Geometry check sheet. Reference: the model listing, model coordinates, mm. Face numbers are marked on the shaded views. A direction names the side the tool comes from. Coordinates: 2 decimals unless noted, no trailing zeros. Write each loop counter-clockwise with the first axis right and the second up, starting at its lowest first coordinate (ties: lowest second). Pieces come first, ordered by that corner, then holes.
from build123d import *
from build123d.topology import SkipClean

# Parameters (mm, degrees)
BOSS_EXTRUDE1_DEPTH = 11.1125
SKETCH3_R           = 17.6
BOSS_EXTRUDE2_DEPTH = 12.7
SKETCH3_5_R         = 11.25
CUT_EXTRUDE2_DEPTH  = 7.5
SKETCH3_6_R         = 9
CUT_EXTRUDE3_DEPTH  = 12.7
BOSS_EXTRUDE3_START = -31.9278
BOSS_EXTRUDE3_DEPTH = 4.953
FILLET1_R           = 1.016
SKETCH5_R           = 1.905
CUT_EXTRUDE4_DEPTH  = 96.510603758
FILLET3_R           = 1.016
CUT_EXTRUDE5_START  = -3.175
CUT_EXTRUDE5_DEPTH  = 3.175
SKETCH9_W           = 10.961249955
SKETCH9_H           = 7.9375
CUT_EXTRUDE6_DEPTH  = 3.175
CUT_EXTRUDE9_DEPTH  = 2.54
SKETCH13_R          = 12.7
SKETCH13_R_2        = 9
BOSS_EXTRUDE6_DEPTH = 3.175
CHAMFER2_SIZE       = 3.175
SKETCH15_R          = 2.54
CUT_EXTRUDE10_DEPTH = 91.477679673


with BuildPart() as part:
    # Sketch2 → Boss-Extrude1 (new, symmetric)
    with BuildSketch(Plane(origin=(0, 0, 0), x_dir=(1, 0, 0), z_dir=(0, 1, 0))):
        Polygon((0, 0), (-57.15, 0), (-84.090768363, -26.940768363), (-76.008537854, -35.022998872), (-53.685538982, -12.7), (0, -12.7), align=None)
        Polygon((57.15, 0), (0, 0), (0, -12.7), (53.685538982, -12.7), (76.008537854, -35.022998872), (84.090768363, -26.940768363), align=None)
    extrude(amount=BOSS_EXTRUDE1_DEPTH, both=True)

    # Sketch3 → Boss-Extrude2 (add)
    with BuildSketch(Plane(origin=(0, 0, 0), x_dir=(-1, 0, 0), z_dir=(0, 0, -1))):
        Circle(SKETCH3_R)
    extrude(amount=-BOSS_EXTRUDE2_DEPTH)

    # Sketch3<5> → Cut-Extrude2 (cut)
    with BuildSketch(Plane(origin=(0, 0, 0), x_dir=(-1, 0, 0), z_dir=(0, 0, -1))):
        Circle(SKETCH3_5_R)
    extrude(amount=-CUT_EXTRUDE2_DEPTH, mode=Mode.SUBTRACT)

    # Sketch3<6> → Cut-Extrude3 (cut)
    with BuildSketch(Plane(origin=(0, 0, 0), x_dir=(-1, 0, 0), z_dir=(0, 0, -1))):
        Circle(SKETCH3_6_R)
    extrude(amount=-CUT_EXTRUDE3_DEPTH, mode=Mode.SUBTRACT)

    # Sketch4 → Boss-Extrude3 (add)
    with BuildSketch(Plane(origin=(55.515768363, 0, 55.515768363), x_dir=(0.707106781186549, 0, -0.707106781186546), z_dir=(0.707106781186546, 0, 0.707106781186549)).offset(BOSS_EXTRUDE3_START)):
        Polygon((27.481152545, -12.6125), (40.411152545, -12.6125), (40.411152545, -11.1125), (28.981152545, -11.1125), (28.981152545, 11.1125), (40.411152545, 11.1125), (40.411152545, 12.6125), (27.481152545, 12.6125), align=None)
    boss_extrude3 = extrude(amount=BOSS_EXTRUDE3_DEPTH)

    # Fillet1
    fillet1_edges = [part.edges().sort_by_distance(p)[0] for p in [
        (66.471505854, -11.1125, 25.485966872),
        (66.471505854, 11.1125, 25.485966872),
    ]]
    fillet(fillet1_edges, radius=FILLET1_R)

    # Sketch5 → Cut-Extrude4 (cut, through all)
    with BuildSketch(Plane(origin=(0, 11.1125, 0), x_dir=(1, 0, 0), z_dir=(0, 1, 0))):
        with BuildLine():
            ThreePointArc((73.278539993, -23.851560258), (73.278539993, -26.545637094), (75.97261683, -26.545637094))
            Line((75.97261683, -26.545637094), (73.278539993, -23.851560258))
        make_face()
        with BuildLine():
            Line((73.278539993, -23.851560258), (75.97261683, -26.545637094))
            ThreePointArc((75.97261683, -26.545637094), (76.385568921, -25.927610614), (76.530578412, -25.198598676))
            ThreePointArc((76.530578412, -25.198598676), (75.35459035, -23.438608166), (73.278539993, -23.851560258))
        make_face()
        with Locations(Location((65.645322291, -16.218342555, 0), (0, 0, 270))):
            Circle(SKETCH5_R)
    cut_extrude4 = extrude(amount=-CUT_EXTRUDE4_DEPTH, mode=Mode.SUBTRACT)

    # Mirror2: Boss-Extrude3, Cut-Extrude4 across plane
    add(boss_extrude3.mirror(Plane(origin=(0, 0, 0), x_dir=(0, 0, 1), z_dir=(1, 0, 0))))
    add(cut_extrude4.mirror(Plane(origin=(0, 0, 0), x_dir=(0, 0, 1), z_dir=(1, 0, 0))), mode=Mode.SUBTRACT)

    # Fillet3
    fillet3_edges = [part.edges().sort_by_distance(p)[0] for p in [
        (-66.471505854, -11.1125, 25.485966872),
        (-66.471505854, 11.1125, 25.485966872),
    ]]
    fillet(fillet3_edges, radius=FILLET3_R)

    # Sketch6 → Cut-Extrude5 (cut)
    with BuildSketch(Plane.XY.offset(12.7).offset(CUT_EXTRUDE5_START)):
        with BuildLine():
            Line((-53.17880895, 11.1125), (-53.17880895, 3.175))
            Line((-53.17880895, 3.175), (-17.311249955, 3.175))
            ThreePointArc((-17.311249955, 3.175), (-15.980371829, 7.374802791), (-13.648162651, 11.1125))
            Line((-13.648162651, 11.1125), (-53.17880895, 11.1125))
        make_face()
        with BuildLine():
            Line((-17.311249955, -3.175), (-53.17880895, -3.175))
            Line((-53.17880895, -3.175), (-53.17880895, -11.1125))
            Line((-53.17880895, -11.1125), (-13.648162651, -11.1125))
            ThreePointArc((-13.648162651, -11.1125), (-15.980371829, -7.374802791), (-17.311249955, -3.175))
        make_face()
        with BuildLine():
            Line((53.17880895, 11.1125), (13.648162651, 11.1125))
            ThreePointArc((13.648162651, 11.1125), (15.980371829, 7.374802791), (17.311249955, 3.175))
            Line((17.311249955, 3.175), (53.17880895, 3.175))
            Line((53.17880895, 3.175), (53.17880895, 11.1125))
        make_face()
        with BuildLine():
            ThreePointArc((17.311249955, -3.175), (15.980371829, -7.374802791), (13.648162651, -11.1125))
            Line((13.648162651, -11.1125), (53.17880895, -11.1125))
            Line((53.17880895, -11.1125), (53.17880895, -3.175))
            Line((53.17880895, -3.175), (17.311249955, -3.175))
        make_face()
    extrude(amount=CUT_EXTRUDE5_DEPTH, mode=Mode.SUBTRACT)

    # Sketch9 → Cut-Extrude6 (cut)
    with SkipClean():  # the faces are left unmerged after this step: merging them gives an invalid solid
        with BuildSketch(Plane(origin=(0, 0, 0), x_dir=(-1, 0, 0), z_dir=(0, 0, -1))):
            with Locations((62.630624978, -7.14375)):
                Rectangle(SKETCH9_W, SKETCH9_H)
            with BuildLine():
                ThreePointArc((17.311249955, -3.175), (15.980371829, -7.374802791), (13.648162651, -11.1125))
                Line((13.648162651, -11.1125), (57.15, -11.1125))
                Line((57.15, -11.1125), (57.15, -3.175))
                Line((57.15, -3.175), (17.311249955, -3.175))
            make_face()
            with BuildLine():
                Line((57.15, 11.1125), (13.648162651, 11.1125))
                ThreePointArc((13.648162651, 11.1125), (15.980371829, 7.374802791), (17.311249955, 3.175))
                Line((17.311249955, 3.175), (57.15, 3.175))
                Line((57.15, 3.175), (57.15, 11.1125))
            make_face()
            with Locations((62.630624978, 7.14375)):
                Rectangle(SKETCH9_W, SKETCH9_H)
            with BuildLine():
                ThreePointArc((-13.648162651, -11.1125), (-15.980371829, -7.374802791), (-17.311249955, -3.175))
                Line((-17.311249955, -3.175), (-57.15, -3.175))
                Line((-57.15, -3.175), (-57.15, -11.1125))
                Line((-57.15, -11.1125), (-13.648162651, -11.1125))
            make_face()
            with Locations((-62.630624978, -7.14375)):
                Rectangle(SKETCH9_W, SKETCH9_H)
            with BuildLine():
                Line((-57.15, 3.175), (-17.311249955, 3.175))
                ThreePointArc((-17.311249955, 3.175), (-15.980371829, 7.374802791), (-13.648162651, 11.1125))
                Line((-13.648162651, 11.1125), (-57.15, 11.1125))
                Line((-57.15, 11.1125), (-57.15, 3.175))
            make_face()
            with Locations((-62.630624978, 7.14375)):
                Rectangle(SKETCH9_W, SKETCH9_H)
        extrude(amount=-CUT_EXTRUDE6_DEPTH, mode=Mode.SUBTRACT)

    # Sketch12 → Cut-Extrude9 (cut)
    with SkipClean():  # the faces are left unmerged after this step: merging them gives an invalid solid
        with BuildSketch(Plane(origin=(55.515768363, 0, 55.515768363), x_dir=(0.7071067811865486, 0, -0.7071067811865465), z_dir=(0.7071067811865465, 0, 0.7071067811865486))):
            with BuildLine():
                Line((28.981152545, 10.0965), (28.981152545, -10.0965))
                ThreePointArc((28.981152545, -10.0965), (29.278732055, -10.81492049), (29.997152545, -11.1125))
                Line((29.997152545, -11.1125), (40.411152545, -11.1125))
                Line((40.411152545, -11.1125), (40.411152545, 11.1125))
                Line((40.411152545, 11.1125), (29.997152545, 11.1125))
                ThreePointArc((29.997152545, 11.1125), (29.278732055, 10.81492049), (28.981152545, 10.0965))
            make_face()
        cut_extrude9 = extrude(amount=-CUT_EXTRUDE9_DEPTH, mode=Mode.SUBTRACT)

    # Mirror3: Cut-Extrude9 across plane
    with SkipClean():  # the faces are left unmerged after this step: merging them gives an invalid solid
        add(cut_extrude9.mirror(Plane(origin=(0, 0, 0), x_dir=(0, 0, 1), z_dir=(1, 0, 0))), mode=Mode.SUBTRACT)

    # Sketch13 → Boss-Extrude6 (add)
    with SkipClean():  # the faces are left unmerged after this step: merging them gives an invalid solid
        with BuildSketch(Plane.XY.offset(12.7)):
            Circle(SKETCH13_R)
            with Locations(Location((0, 0, 0), (0, 0, 180))):
                Circle(SKETCH13_R_2, mode=Mode.SUBTRACT)
        extrude(amount=BOSS_EXTRUDE6_DEPTH)

    # Chamfer2
    chamfer2_edges = [part.edges().sort_by_distance(p)[0] for p in [
        (53.17880895, 7.14375, 9.525),
        (53.17880895, -7.14375, 9.525),
        (-53.17880895, 7.14375, 9.525),
        (-53.17880895, -7.14375, 9.525),
    ]]
    chamfer(chamfer2_edges, length=CHAMFER2_SIZE - 0.0001)  # a hair under: the kernel refuses the full size

    # Sketch15 → Cut-Extrude10 (cut, through all)
    with BuildSketch(Plane(origin=(0, 0, 0), x_dir=(-1, 0, 0), z_dir=(0, 0, -1))):
        with Locations((21.59, 0)):
            Circle(SKETCH15_R)
        with Locations(Location((-21.59, 0, 0), (0, 0, 180))):
            Circle(SKETCH15_R)
    extrude(amount=-CUT_EXTRUDE10_DEPTH, mode=Mode.SUBTRACT)


solid = part.part
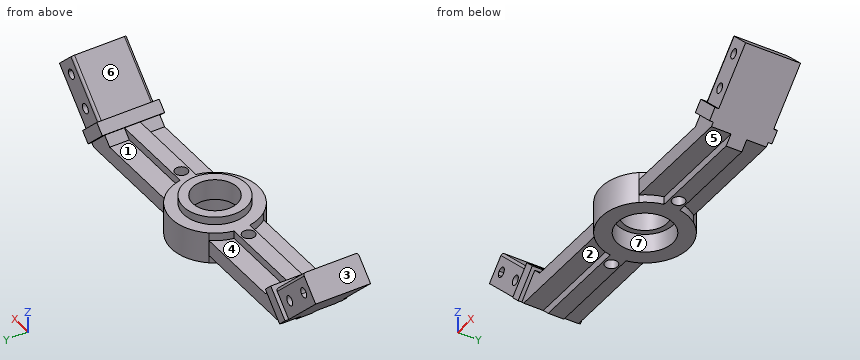
1. Sectioned sample at A-A, the plane x = 21.59. Record the boundary of the cut face in (y, z) (1 decimal), and give its area (3 significant figures).
Computed values:
outline: (-11.1, 3.2) - (-3.2, 3.2) - (-3.2, 0) - (-2.5, 0) - (-2.5, 12.7) - (-3.2, 12.7) - (-3.2, 9.5) - (-11.1, 9.5) - close; (2.5, 0) - (3.2, 0) - (3.2, 3.2) - (11.1, 3.2) - (11.1, 9.5) - (3.2, 9.5) - (3.2, 12.7) - (2.5, 12.7) - close
area: 117 mm2
2. Sectioned sample at D-D, the plane x = 0. Record the boundary of the cut face in (y, z) (3 decimals).
Computed values:
outline: (-17.6, 0) - (-11.25, 0) - (-11.25, 7.5) - (-9, 7.5) - (-9, 15.875) - (-12.7, 15.875) - (-12.7, 12.7) - (-17.6, 12.7) - close; (9, 7.5) - (11.25, 7.5) - (11.25, 0) - (17.6, 0) - (17.6, 12.7) - (12.7, 12.7) - (12.7, 15.875) - (9, 15.875) - close
3. Access from +Z, -Z, +X, -X, +Y, -Y to the whole of each face (thin tool, end or side, straight path). Record for the marked faces 4, 5, 6 and 7.
Computed values:
face 4: +Z, +Y
face 5: -Z, +X, -Y
face 6: +Z, +Y, -Y
face 7: -Z
4. Gauge pin test, flat ends, axial feed: pin 1 Ø8 at (y, z) = (-6.5, 25) entering from +X; pin 2 Ø1.5 at (y, z) = (13, 12.5) entering from +X; pin 3 Ø5 at (x, z) = (38, 10) entering from -Y. Record the tip position at first contact, or that the pin passes through.
Computed values:
pin 1: stops at x = 82.29
pin 2: stops at x = 61.03
pin 3: stops at y = -11.11
5. Sectioned sample at C-C, the plane y = 6. Give the number of separate pieces and of enclosed holes in the cut face, and give its area (3 significant figures).
Computed values:
separate pieces: 2
enclosed holes: 4
area: 1,440 mm2
6. Thickness scan on line 1 along Y through (x, z) = (0, 2.5); line 2 along X through (y, z) = (5, 24); line 3 along Y through (x, z) = (0, 10). Record the ranges inside material, lowest first.
Computed values:
line 1: y = -17.6 to -11.25, 11.25 to 17.6
line 2: x = -81.15 to -76.11, -73.14 to -64.99, 64.99 to 73.14, 76.11 to 81.15
line 3: y = -17.6 to -9, 9 to 17.6
7. Sectioned sample at B-B, the plane x = -39. Record the boundary of the cut face in (y, z) (1 decimal).
Computed values:
outline: (-11.1, 3.2) - (-3.2, 3.2) - (-3.2, 0) - (3.2, 0) - (3.2, 3.2) - (11.1, 3.2) - (11.1, 9.5) - (3.2, 9.5) - (3.2, 12.7) - (-3.2, 12.7) - (-3.2, 9.5) - (-11.1, 9.5) - close
8. Draft check along X on the marked faces 1, 2 and 3. Enter one of: released by +X, released by -X, zero draft, split by the parting line, or undercut.
Computed values:
face 1: undercut
face 2: zero draft
face 3: released by -X
